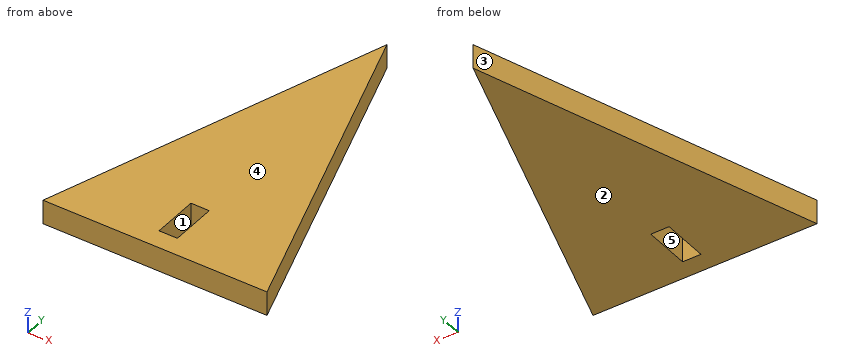
```python
from build123d import *

# Parameters (mm, degrees)
SKETCH2_W           = 2.413
SKETCH2_H           = 6.096
BOSS_EXTRUDE1_DEPTH = 3.175


with BuildPart() as part:
    # Sketch2 → Boss-Extrude1 (new body)
    with BuildSketch(Plane.XY):
        Polygon((-16.084625597, -40.368802078), (-1.352625597, 4.081197922), (13.379374403, -40.368802078), align=None)
        with Locations((-1.352625597, -34.780802078)):
            Rectangle(SKETCH2_W, SKETCH2_H, mode=Mode.SUBTRACT)
    extrude(amount=BOSS_EXTRUDE1_DEPTH)


solid = part.part
```
The model under review builds one solid part; all positions refer to its coordinate system, in mm. Face numbers are marked on the shaded views. A direction names the side the tool comes from. Round coordinates to 2 decimals unless told otherwise and drop trailing zeros. Write each loop counter-clockwise with the first axis right and the second up, starting at its lowest first coordinate (ties: lowest second). Pieces come first, ordered by that corner, then holes. Notation, with made-up numbers: (16.5, -7) - (57.5, -7) arc R25 ccw to (57.5, 21) - close; hole circle Ø10 at (46.25, -18). An arc over 180 degrees is marked (long way). Answer as CSV lines item,"result". Start each with the question number.
(1) For the marked faces 1 and 2, list the 3-axis set-ups (+Z, -Z, +X, -X, +Y, -Y) from which the entire face can be reached by the end or side of a thin tool; tool diameter is ignored.
(2) We need section C-C on x = -6.5. State the section outline as (y, z) points (3 decimals), plus the area to 3 significant figures.
(3) We need section A-A on z = 1.9. State the section outline as (x, y) points.
(4) We need section B-B on y = -32.5. State the section outline as (x, z) points (3 decimals).
(5) Draft analysis for pull direction X (two halves, no side actions). For the marked faces 3, 4 and 5, state which applies: pulls with the +X half, pulls with the -X half, needs draft (parallel to the pull), parting line crosses it, or undercut.
(6) For pin 1 Ø1 at (y, z) = (-34.5, 2) entering from -X; pin 2 Ø1 at (x, y) = (-4.5, -1.5) entering from +Z, all flat-tipped, find the tip position at first contact; note any pin that passes through.
(7) We need section D-D on y = 0. State the section outline as (x, z) points (3 decimals), plus the area to 3 significant figures.
(8) To check wall thickness, follow line 1 (X direction, y = -34, z = 1.5); line 2 (X direction, y = -37.5, z = 0.4); line 3 (X direction, y = -7, z = 1.35). State the ranges of each line that lie inside material, in increasing order.
Worked answers:
1,face 1,"+Z, -Z"
1,face 2,"-Z, +X, -X, +Y, -Y"
2,outline,"(-40.369, 0) - (-11.45, 0) - (-11.45, 3.175) - (-40.369, 3.175) - close"
2,area,"91.8 mm²"
3,outline,"(-16.08, -40.37) - (13.38, -40.37) - (-1.35, 4.08) - close; hole (-2.56, -37.83) - (-0.15, -37.83) - (-0.15, -31.73) - (-2.56, -31.73) - close"
4,outline,"(-13.477, 0) - (-2.559, 0) - (-2.559, 3.175) - (-13.477, 3.175) - close; (-0.146, 0) - (10.771, 0) - (10.771, 3.175) - (-0.146, 3.175) - close"
5,face 3,"pulls with the -X half"
5,face 4,"needs draft"
5,face 5,"undercut"
6,pin 1,"x = -14.31"
6,pin 2,"through"
7,outline,"(-2.705, 0) - (0, 0) - (0, 3.175) - (-2.705, 3.175) - close"
7,area,"8.59 mm²"
8,line 1,"-13.97 to -2.56, -0.15 to 11.27"
8,line 2,"-15.13 to -2.56, -0.15 to 12.43"
8,line 3,"-5.03 to 2.32"
